Source: CAD feature listing. Evaluate the final solid. Frame: model axes, mm. Face numbers are marked on the shaded views. A direction names the side the tool comes from. Coordinates: 2 decimals unless noted, no trailing zeros. Order: outer loops, then holes, each group sorted by start corner. A loop starts at its lowest first (then second) coordinate and runs counter-clockwise, first axis right, second up.
```python
from build123d import *

# Parameters (mm, degrees)
SKETCH1_W           = 70
SKETCH1_H           = 50
BOSS_EXTRUDE1_DEPTH = 50
CUT_EXTRUDE1_DEPTH  = 50
CUT_EXTRUDE3_DEPTH  = 30
BOSS_EXTRUDE2_DEPTH = 30
SKETCH6_W           = 70
SKETCH6_H           = 50
CUT_EXTRUDE4_DEPTH  = 30
BOSS_EXTRUDE3_DEPTH = 30
SKETCH8_W           = 30
SKETCH8_H           = 10
CUT_EXTRUDE6_DEPTH  = 15
BOSS_EXTRUDE4_DEPTH = 15
BOSS_EXTRUDE5_DEPTH = 15
SKETCH11_W          = 15
SKETCH11_H          = 10
CUT_EXTRUDE8_DEPTH  = 30


with BuildPart() as part:
    # Sketch1 → Boss-Extrude1 (new body)
    with BuildSketch(Plane.XY):
        with Locations((35, 25)):
            Rectangle(SKETCH1_W, SKETCH1_H)
    extrude(amount=BOSS_EXTRUDE1_DEPTH)

    # Sketch2 → Cut-Extrude1 (cut)
    with BuildSketch(Plane.XY.offset(50)):
        Polygon((0, 20), (30, 50), (0, 50), align=None)
    extrude(amount=-CUT_EXTRUDE1_DEPTH, mode=Mode.SUBTRACT)

    # Sketch3 → Cut-Extrude3 (cut)
    with BuildSketch(Plane.XY.offset(50)):
        Polygon((0, 0), (40, 40), (40, 50), (30, 50), (0, 20), align=None)
    extrude(amount=-CUT_EXTRUDE3_DEPTH, mode=Mode.SUBTRACT)

    # Sketch4 → Boss-Extrude2 (add)
    with BuildSketch(Plane(origin=(-13.636363636, 13.636363636, 9.090909091), x_dir=(0.768706115, 0.532181156, 0.354787438), z_dir=(-0.639602149, 0.639602149, 0.426401433))):
        Polygon((17.73937188, -5.547001962), (17.73937188, -41.602514717), (69.774862727, -19.414506868), (56.765990015, 11.094003925), align=None)
    extrude(amount=-BOSS_EXTRUDE2_DEPTH)

    # Sketch6 → Cut-Extrude4 (cut)
    with BuildSketch(Plane.XZ):
        with Locations((35, 25)):
            Rectangle(SKETCH6_W, SKETCH6_H)
    extrude(amount=CUT_EXTRUDE4_DEPTH, mode=Mode.SUBTRACT)

    # Sketch7 → Boss-Extrude3 (add)
    with BuildSketch(Plane.ZY):
        Polygon((20, 20), (20, 0), (50, 0), align=None)
    extrude(amount=-BOSS_EXTRUDE3_DEPTH)

    # Sketch8 → Cut-Extrude6 (cut)
    with BuildSketch(Plane.XY.offset(50)):
        with Locations((55, 45)):
            Rectangle(SKETCH8_W, SKETCH8_H)
    extrude(amount=-CUT_EXTRUDE6_DEPTH, mode=Mode.SUBTRACT)

    # Sketch9 → Boss-Extrude4 (add)
    with BuildSketch(Plane(origin=(-13.636363636, 13.636363636, 9.090909091), x_dir=(-0.768706115, -0.532181156, -0.354787438), z_dir=(0.639602149, -0.639602149, -0.426401433))):
        Polygon((-56.765990015, 11.094003925), (-69.774862727, -19.414506868), (-69.774862727, -1.386750491), align=None)
    extrude(amount=BOSS_EXTRUDE4_DEPTH)

    # Sketch10 → Boss-Extrude5 (add)
    with BuildSketch(Plane(origin=(0, 50, 0), x_dir=(1, 0, 0), z_dir=(0, 1, 0))):
        Polygon((30, -20), (40, -20), (40, -35), align=None)
    extrude(amount=-BOSS_EXTRUDE5_DEPTH)

    # Sketch11 → Cut-Extrude8 (cut)
    with BuildSketch(Plane(origin=(70, 0, 0), x_dir=(0, 0, -1), z_dir=(1, 0, 0))):
        with Locations((-42.5, 45)):
            Rectangle(SKETCH11_W, SKETCH11_H)
    extrude(amount=-CUT_EXTRUDE8_DEPTH, mode=Mode.SUBTRACT)


solid = part.part
```
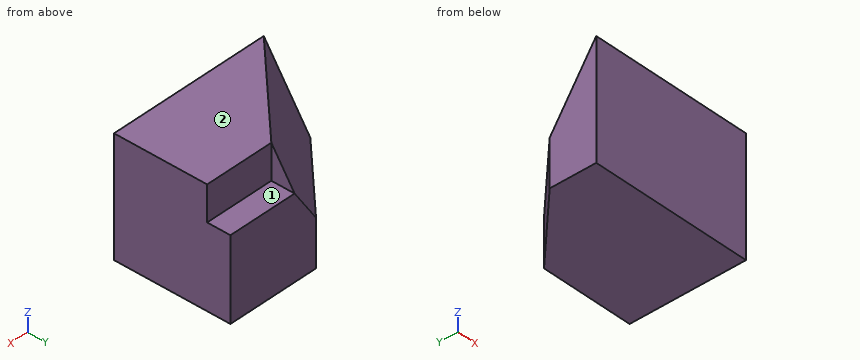
1. Access query for the marked faces 1 and 2. Directions: +Z, -Z, +X, -X, +Y, -Y. A direction counts if a zero-diameter tool reaches every point of the face in a straight line with its end or side. Return the directions, or none.
Findings:
face 1: +Z, +X, +Y
face 2: +Z, +X, -X, +Y, -Y
2. Ray query, line 1 (Z direction, x = 67.5, y = 44.5); line 2 (Y direction, x = 43.5, z = 35.5); line 3 (X direction, y = 21.5, z = 34.5). Return the intervals inside material, ascending.
Findings:
line 1: z = 0 to 35
line 2: y = 0 to 40
line 3: x = 11.17 to 70
3. Section query C-C on x = 56.5. Return loops of the section in (y, z), plus the area to 3 significant figures.
Findings:
outline: (0, 0) - (50, 0) - (50, 35) - (40, 35) - (40, 50) - (0, 50) - close
area: 2,350 mm2
4. Pin query (flat end, axial travel): P1, Ø4, axis at x = 28.5, z = 36.5, coming from the +Y side; P2, Ø3, axis at x = 15, y = 24.5, coming from the +Z side; P3, Ø7.5, axis at x = 59, z = 45.5, coming from the +Y side. Return the tip coordinate at first contact, or that it passes through.
Findings:
P1: stops at y = 39.9
P2: stops at z = 38.93
P3: stops at y = 40
5. Section query D-D on y = 34. Return loops of the section in (x, z), plus the area to 3 significant figures.
Findings:
outline: (14, 0) - (70, 0) - (70, 50) - (34, 50) - (14, 20) - close
area: 2,500 mm2
6. Section query B-B on y = 46. Return loops of the section in (x, z), plus the area to 3 significant figures.
Findings:
outline: (26, 0) - (70, 0) - (70, 35) - (40, 35) - (40, 41) - (26, 20) - close
area: 1,480 mm2
7. Section query A-A on z = 7. Return loops of the section in (x, y).
Findings:
outline: (0, 0) - (70, 0) - (70, 50) - (30, 50) - (0, 20) - close
